```python
from build123d import *

# Parameters (mm, degrees)
BOSS_EXTRUDE1_DEPTH = 4
SKETCH2_R           = 3
BOSS_EXTRUDE2_DEPTH = 2
SKETCH3_R           = 1.3
CUT_EXTRUDE1_DEPTH  = 6
SKETCH4_R           = 2.6
BOSS_EXTRUDE3_DEPTH = 4
FILLET1_R           = 3
FILLET2_R           = 2
SKETCH5_R           = 1.625
CUT_EXTRUDE2_DEPTH  = 10


with BuildPart() as part:
    # Sketch1 → Boss-Extrude1 (new body)
    with BuildSketch(Plane(origin=(0, 0, 0), x_dir=(1, 0, 0), z_dir=(0, 1, 0))):
        with BuildLine():
            Line((3, 0), (107, 0))
            ThreePointArc((107, 0), (109.121320344, 0.878679656), (110, 3))
            Line((110, 3), (110, 87))
            ThreePointArc((110, 87), (109.121320344, 89.121320344), (107, 90))
            Line((107, 90), (3, 90))
            ThreePointArc((3, 90), (0.878679656, 89.121320344), (0, 87))
            Line((0, 87), (0, 3))
            ThreePointArc((0, 3), (0.878679656, 0.878679656), (3, 0))
        make_face()
    extrude(amount=BOSS_EXTRUDE1_DEPTH)

    # Sketch2 → Boss-Extrude2 (add)
    with BuildSketch(Plane(origin=(0, 4, 0), x_dir=(1, 0, 0), z_dir=(0, 1, 0))):
        with Locations(Location((22, 72, 0), (0, 0, 270))):
            Circle(SKETCH2_R)
        with Locations(Location((103.28, 23.74, 0), (0, 0, 270))):
            Circle(SKETCH2_R)
        with Locations(Location((96.93, 72, 0), (0, 0, 270))):
            Circle(SKETCH2_R)
        with Locations(Location((20, 23.74, 0), (0, 0, 270))):
            Circle(SKETCH2_R)
    extrude(amount=BOSS_EXTRUDE2_DEPTH)

    # Sketch3 → Cut-Extrude1 (cut)
    with BuildSketch(Plane(origin=(0, 6, 0), x_dir=(1, 0, 0), z_dir=(0, 1, 0))):
        with Locations(Location((22, 72, 0), (0, 0, 270))):
            Circle(SKETCH3_R)
        with Locations(Location((96.93, 72, 0), (0, 0, 270))):
            Circle(SKETCH3_R)
        with Locations(Location((103.28, 23.74, 0), (0, 0, 270))):
            Circle(SKETCH3_R)
        with Locations(Location((20, 23.74, 0), (0, 0, 270))):
            Circle(SKETCH3_R)
    extrude(amount=-CUT_EXTRUDE1_DEPTH, mode=Mode.SUBTRACT)

    # Sketch4 → Boss-Extrude3 (add)
    with BuildSketch(Plane(origin=(0, 0, -90), x_dir=(-1, 0, 0), z_dir=(0, 0, -1))):
        with BuildLine():
            Line((-107, 0), (-3, 0))
            Line((-3, 0), (-3, 17))
            ThreePointArc((-3, 17), (-3.878679656, 19.121320344), (-6, 20))
            Line((-6, 20), (-104, 20))
            ThreePointArc((-104, 20), (-106.121320344, 19.121320344), (-107, 17))
            Line((-107, 17), (-107, 0))
        make_face()
        with Locations((-82, 15)):
            Circle(SKETCH4_R, mode=Mode.SUBTRACT)
        with Locations((-28, 15)):
            Circle(SKETCH4_R, mode=Mode.SUBTRACT)
    extrude(amount=BOSS_EXTRUDE3_DEPTH)

    # Fillet1
    # the kernel refuses this fillet: 3 mm, written as the material it adds along each edge
    with BuildSketch(Plane(origin=(3, 0, -90), x_dir=(-0.9659258262890682, 0, 0.25881904510252113), z_dir=(0, 1, 0))) as fillet1_piece_1:
        with BuildLine():
            CenterArc((2.329371406, -2.897777479), FILLET1_R, 105, 60)
            Line((-0.568406073, -2.121320344), (0, 0))
            ThreePointArc((0, 0), (0.776457135, -0.102222521), (1.552914271, 0))
        make_face()
    extrude(amount=4)
    with BuildSketch(Plane(origin=(107, 0, -90), x_dir=(0.9659258262890682, 0, 0.2588190451025207), z_dir=(0, 1, 0))) as fillet1_piece_2:
        with BuildLine():
            CenterArc((2.329371406, 2.897777479), FILLET1_R, 195, 60)
            Line((-0.568406073, 2.121320344), (0, 0))
            ThreePointArc((0, 0), (0.776457135, 0.102222521), (1.552914271, 0))
        make_face()
    extrude(amount=4)

    # Fillet2
    fillet2_edges = [part.edges().sort_by_distance(p)[0] for p in [
        (55, 4, -90),
    ]]
    fillet(fillet2_edges, radius=FILLET2_R)

    # Sketch5 → Cut-Extrude2 (cut)
    with BuildSketch(Plane(origin=(0, 4, 0), x_dir=(1, 0, 0), z_dir=(0, 1, 0))):
        with Locations(Location((5, 85, 0), (0, 0, 270))):
            Circle(SKETCH5_R)
        with Locations(Location((105, 85, 0), (0, 0, 270))):
            Circle(SKETCH5_R)
        with Locations(Location((105, 5, 0), (0, 0, 270))):
            Circle(SKETCH5_R)
        with Locations(Location((5, 5, 0), (0, 0, 270))):
            Circle(SKETCH5_R)
    extrude(amount=-CUT_EXTRUDE2_DEPTH, mode=Mode.SUBTRACT)


solid = part.part
```
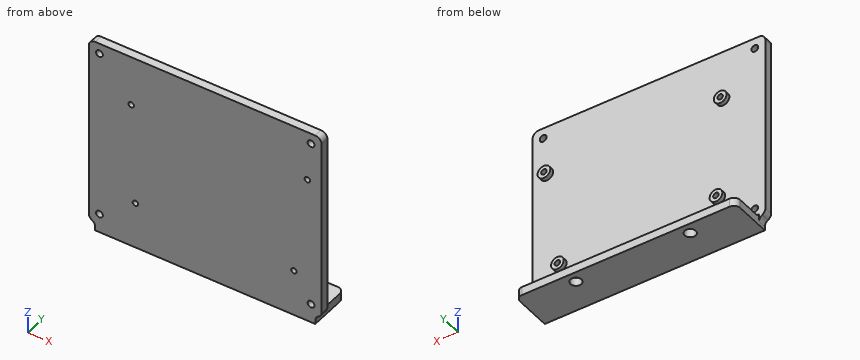
The model under review builds one solid part; all positions refer to its coordinate system, in mm. Coordinates: 2 decimals unless noted, no trailing zeros. Write each loop counter-clockwise with the first axis right and the second up, starting at its lowest first coordinate (ties: lowest second). Pieces come first, ordered by that corner, then holes.
1) We need section B-B on x = 28. State the section outline as (y, z) points.
2) Clearance check with flat-ended pins moving along their axes: pin 1 Ø5 at (x, z) = (78, -60) entering from +Y; pin 2 Ø3 at (x, z) = (98, -72.5) entering from +Y; pin 3 Ø7 at (x, y) = (60, 12.5) entering from +Z. State where each tip first meets the part, or that it passes through.
3) We need section A-A on z = -85. State the section outline as (x, y) points (3 decimals).
4) We need section D-D on y = 8.75. State the section outline as (x, z) points, then the cut area to 3 significant figures.
5) We need section C-C on x = 89. State the section outline as (y, z) points.
6) To check wall thickness, follow probe 1 along Z at (x, y) = (105, 1.6) (3 decimals); probe 2 along X at (y, z) = (2.4, -23.74); probe 3 along X at (y, z) = (1.5, -85) (3 decimals). State the ranges of each line that lie inside material, in increasing order.
Answer list:
1. outline: (0, -94) - (12.4, -94) - (12.4, -90) - (6, -90) arc R2 cw to (4, -88) - (4, 0) - (0, 0) - close; (17.6, -94) - (20, -94) - (20, -90) - (17.6, -90) - close
2. pin 1: stops at y = 4
2. pin 2: stops at y = 6
2. pin 3: stops at z = -90
3. outline: (0, 0) - (3.375, 0) - (3.375, 4) - (0, 4) - close; (6.625, 0) - (103.375, 0) - (103.375, 4) - (6.625, 4) - close; (106.625, 0) - (110, 0) - (110, 4) - (106.625, 4) - close
4. outline: (3, -94) - (107, -94) - (107, -90) - (3, -90) - close
4. area: 416 mm2
5. outline: (0, -94) - (20, -94) - (20, -90) - (6, -90) arc R2 cw to (4, -88) - (4, 0) - (0, 0) - close
6. probe 1: z = -94 to -86.625, -83.375 to -6.625, -3.375 to 0
6. probe 2: x = 0 to 18.7, 21.3 to 101.98, 104.58 to 110
6. probe 3: x = 0 to 3.375, 6.625 to 103.375, 106.625 to 110
